For this review, take the finished solid that the model builds, in its own axes (mm). Face numbers are marked on the shaded views. A direction names the side the tool comes from. Coordinates: 2 decimals unless noted, no trailing zeros. Write each loop counter-clockwise with the first axis right and the second up, starting at its lowest first coordinate (ties: lowest second). Pieces come first, ordered by that corner, then holes. Notation, with made-up numbers: (1.5, 48.25) -> (45.5, 48.25) arc R22 ccw to (45.5, 86.25) -> close; hole circle Ø10 at (59, -24.75). An arc over 180 degrees is marked (long way). Put each result on its own line as item: value. Start each with the question number.
Item 1: For the marked faces 1 and 2, list the 3-axis set-ups (+Z, -Z, +X, -X, +Y, -Y) from which the entire face can be reached by the end or side of a thin tool; tool diameter is ignored.
Item 2: To check wall thickness, follow L1, parallel to Z at x = -18, y = 0; L2, parallel to Z at x = -8.5, y = 1; L3, parallel to X at y = 36.5, z = -24. State the ranges of each line that lie inside material, in increasing order.
Item 3: Consider section A-A on z = 0. Give the number of separate pieces and of enclosed holes in the cut face, and give its area (3 significant figures).
Item 4: Consider section B-B on y = 53. Give the boundary of the cut face in (x, z), and give its area (3 significant figures).
Item 5: Insertion check: P1, Ø12, axis at x = 47.5, z = 20.5, coming from the +Y side; P2, Ø5, axis at x = -40.5, z = 3, coming from the +Y side; P3, Ø2, axis at x = 2, y = 2, coming from the -Z side. Each pin has a flat end and moves straight along its axis. Give the tip position at first contact, or say it passes through.
Item 6: The part is to be moulded in two halves that separate along Y. For the marked faces 3 and 4, say which applies: +Y half, -Y half, draft (parallel to the pull), parting line (faces both ways), or undercut.
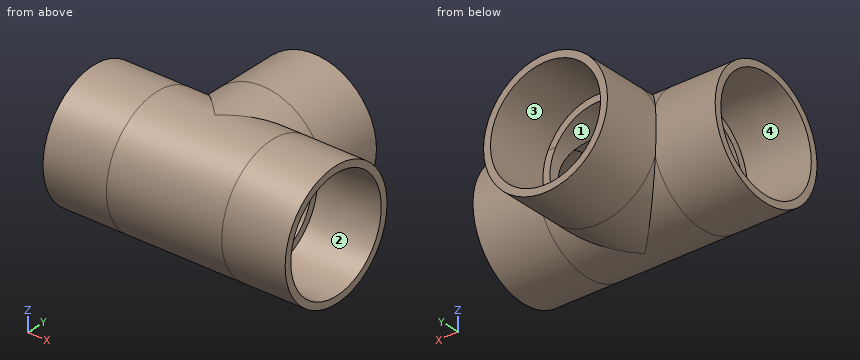
```python
from build123d import *

# Parameters (mm, degrees)
BOSS_EXTRUDE1_DEPTH = 63.5
BOSS_EXTRUDE2_REACH = 67.881
SKETCH5_R           = 26.2509
CUT_EXTRUDE1_DEPTH  = 63.5
CUT_EXTRUDE2_START  = -31.75
SKETCH6_R           = 26.2509
CUT_EXTRUDE2_DEPTH  = 31.75


with BuildPart() as part:
    # Sketch1 → Revolve1 (revolve)
    with BuildSketch(Plane.XY):
        Polygon((-66.675, -34.13125), (-31.75, -34.13125), (-31.75, -30.0863), (-66.675, -30.3149), align=None)
    revolve(axis=Axis((-66.675, 0, 0), (1, 0, 0)))


with BuildPart() as body_2:
    # Mirror1: mirrored copy
    add(part.part.mirror(Plane(origin=(0, 0, 0), x_dir=(0, 0, 1), z_dir=(1, 0, 0))))


with BuildPart() as body_3:
    # Sketch2 → Revolve2 (revolve)
    with BuildSketch(Plane.XY):
        Polygon((30.3149, 66.675), (30.0863, 31.75), (34.13125, 31.75), (34.13125, 66.675), align=None)
    revolve(axis=Axis((0, 0, 0), (0, 1, 0)))


with BuildPart() as part_1:
    add(part.part)

    add(body_2.part)  # Boss-Extrude1 merges body 2

    add(body_3.part)  # Boss-Extrude1 merges body 3
    # Sketch3 → Boss-Extrude1 (add)
    with BuildSketch(Plane(origin=(-31.75, 0, 0), x_dir=(0, 0, -1), z_dir=(1, 0, 0))):
        with BuildLine():
            Line((12.525163734, 31.75), (-12.525163734, 31.75))
            ThreePointArc((-12.525163734, 31.75), (0, -34.13125), (12.525163734, 31.75))
        make_face()
    extrude(amount=BOSS_EXTRUDE1_DEPTH)

    # Sketch4 → Boss-Extrude2 (add, up to next)
    with BuildSketch(Plane.XZ.offset(-31.75), mode=Mode.PRIVATE) as boss_extrude2_sk1:
        with BuildLine():
            ThreePointArc((-31.75, -12.525163734), (0, -34.13125), (31.75, -12.525163734))
            Line((31.75, -12.525163734), (-31.75, -12.525163734))
        make_face()
    boss_extrude2_tool1 = extrude(boss_extrude2_sk1.sketch, amount=BOSS_EXTRUDE2_REACH, mode=Mode.PRIVATE) - part_1.part
    add(boss_extrude2_tool1.solids().sort_by_distance((0, 31.75, -21.455636))[0])
    # Sketch4 → Boss-Extrude2 (add, up to next)
    with BuildSketch(Plane.XZ.offset(-31.75), mode=Mode.PRIVATE) as boss_extrude2_sk2:
        with BuildLine():
            ThreePointArc((31.75, 12.525163734), (0, 34.13125), (-31.75, 12.525163734))
            Line((-31.75, 12.525163734), (31.75, 12.525163734))
        make_face()
    boss_extrude2_tool2 = extrude(boss_extrude2_sk2.sketch, amount=BOSS_EXTRUDE2_REACH, mode=Mode.PRIVATE) - part_1.part
    add(boss_extrude2_tool2.solids().sort_by_distance((0, 31.75, 21.455636))[0])

    # Sketch5 → Cut-Extrude1 (cut)
    with BuildSketch(Plane.ZY.offset(31.75)):
        Circle(SKETCH5_R)
    extrude(amount=-CUT_EXTRUDE1_DEPTH, mode=Mode.SUBTRACT)

    # Sketch6 → Cut-Extrude2 (cut)
    with BuildSketch(Plane(origin=(0, 31.75, 0), x_dir=(1, 0, 0), z_dir=(0, 1, 0)).offset(CUT_EXTRUDE2_START)):
        Circle(SKETCH6_R)
    extrude(amount=CUT_EXTRUDE2_DEPTH, mode=Mode.SUBTRACT)


solid = part_1.part
```
Return value:
1. face 1: +Y
1. face 2: +X
2. L1: -34.13 to -26.25, 26.25 to 34.13
2. L2: -34.12 to -26.23, 26.23 to 34.12
2. L3: -24.27 to -18.19, 18.19 to 24.27
3. separate pieces: 3
3. enclosed holes: 0
3. area: 1,370 mm^2
4. outline: circle Ø68.26 at (0, 0); hole circle Ø60.45 at (0, 0)
4. area: 790 mm^2
5. P1: y = 30.9
5. P2: y = 34.13
5. P3: z = -34.12
6. face 3: +Y half
6. face 4: undercut
